```python
from build123d import *

# Parameters (mm, degrees)
F0_W     = 45
F0_H     = 15
F1_DEPTH = 20
F2_W     = 43
F2_H     = 11
F3_DEPTH = 15
F5_START = -2
F5_DEPTH = 11


with BuildPart() as f1:
    # F0 (on Top) → F1 (new body)
    with BuildSketch(Plane.XY):
        Rectangle(F0_W, F0_H)
    extrude(amount=F1_DEPTH)

    # F2 (on face) → F3 (cut)
    with BuildSketch(Plane.XY.offset(20)):
        with Locations((1, 0)):
            Rectangle(F2_W, F2_H)
    extrude(amount=-F3_DEPTH, mode=Mode.SUBTRACT)

    # F4 (on face) → F5 (cut)
    with BuildSketch(Plane.XZ.offset(7.5).offset(F5_START)):
        Polygon((22.5, 5), (-20.5, 5), (22.5, 2), align=None)
    extrude(amount=-F5_DEPTH, mode=Mode.SUBTRACT)


solid = f1.part
```
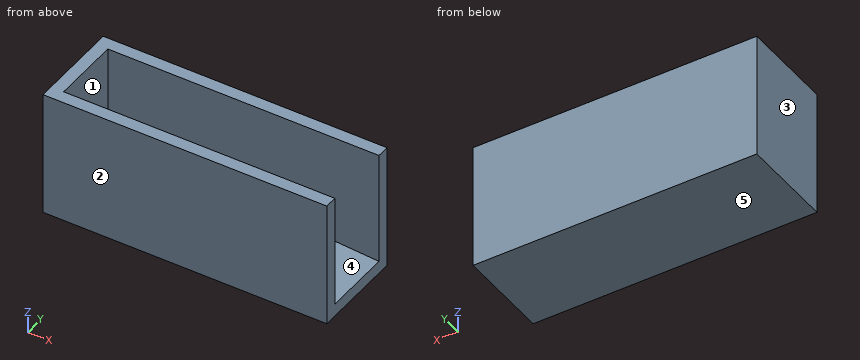
Geometry check sheet. Reference: the model listing, model coordinates, mm. Face numbers are marked on the shaded views. A direction names the side the tool comes from. Round coordinates to 2 decimals unless told otherwise and drop trailing zeros. Write each loop counter-clockwise with the first axis right and the second up, starting at its lowest first coordinate (ties: lowest second). Pieces come first, ordered by that corner, then holes. Notation, with made-up numbers: (-30.5, -35.75) -> (6.5, -35.75) arc R32 cw to (6.5, -9.75) -> close; hole circle Ø4 at (49, 64.25). An arc over 180 degrees is marked (long way). Put each result on its own line as item: value.
1) Cross-section at B-B, the plane x = 16. Enter the section's corners in (y, z).
Recorded:
outline: (-7.5, 0) -> (7.5, 0) -> (7.5, 20) -> (5.5, 20) -> (5.5, 2.45) -> (-5.5, 2.45) -> (-5.5, 20) -> (-7.5, 20) -> close
2) Cross-section at A-A, the plane z = 6.25. Enter the section's corners in (x, y), plus the area to 3 significant figures.
Recorded:
outline: (-22.5, -7.5) -> (22.5, -7.5) -> (22.5, -5.5) -> (-20.5, -5.5) -> (-20.5, 5.5) -> (22.5, 5.5) -> (22.5, 7.5) -> (-22.5, 7.5) -> close
area: 202 mm2
3) Depth check by flat-ended pin: P1, Ø4, axis at y = 2.5, z = 12, coming from the +X side. Enter the tip coordinate at first touch or a pass-through.
Recorded:
P1: stops at x = -20.5
4) Release check for a two-part mould opening along Y. For the marked faces 1, 2 and 3 record: pulls with the +Y half, pulls with the -Y half, needs draft (parallel to the pull), parting line crosses it, or undercut.
Recorded:
face 1: undercut
face 2: pulls with the -Y half
face 3: needs draft
5) Access from +Z, -Z, +X, -X, +Y, -Y to the whole of each face (thin tool, end or side, straight path). Record for the marked faces 4 and 5.
Recorded:
face 4: +Z, +X
face 5: -Z, +X, -X, +Y, -Y
6) Cross-section at C-C, the plane y = -2. Enter the section's corners in (x, z).
Recorded:
outline: (-22.5, 0) -> (22.5, 0) -> (22.5, 2) -> (-20.5, 5) -> (-20.5, 20) -> (-22.5, 20) -> close
7) Thickness scan on probe 1 along Y at (x, z) = (3.5, 15.75); probe 2 along X at (y, z) = (-0.5, 18); probe 3 along Z at (x, y) = (-14.5, 4.75). Record the ranges inside material, lowest first. Write a range as from..to.
Recorded:
probe 1: y = -7.5..-5.5, 5.5..7.5
probe 2: x = -22.5..-20.5
probe 3: z = 0..4.58
